```python
from build123d import *

# Parameters (mm, degrees)
SKETCH1_W           = 101.6
SKETCH1_H           = 101.6
SKETCH1_R           = 12.7
BOSS_EXTRUDE1_DEPTH = 3.175
SKETCH2_R           = 23.495
CUT_EXTRUDE1_DEPTH  = 5.08


with BuildPart() as part:
    # Sketch1 → Boss-Extrude1 (new body, symmetric)
    with BuildSketch(Plane(origin=(0, 0, 0), x_dir=(1, 0, 0), z_dir=(0, 1, 0))):
        Rectangle(SKETCH1_W, SKETCH1_H)
        with Locations((-31.75, 31.75)):
            Circle(SKETCH1_R, mode=Mode.SUBTRACT)
        with Locations((31.75, 31.75)):
            Circle(SKETCH1_R, mode=Mode.SUBTRACT)
    extrude(amount=BOSS_EXTRUDE1_DEPTH, both=True)

    # Sketch2 → Cut-Extrude1 (cut)
    with BuildSketch(Plane(origin=(0, 3.175, 0), x_dir=(1, 0, 0), z_dir=(0, 1, 0))):
        with Locations((-25.4, -10.318450471)):
            Circle(SKETCH2_R)
        with Locations((25.4, -10.318450471)):
            Circle(SKETCH2_R)
    extrude(amount=-CUT_EXTRUDE1_DEPTH, mode=Mode.SUBTRACT)


solid = part.part
```
Geometry check sheet. Reference: the model listing, model coordinates, mm. A direction names the side the tool comes from. Round coordinates to 2 decimals unless told otherwise and drop trailing zeros. Loops run counter-clockwise (first coordinate to the right, second up) from the corner with the lowest first, then second, coordinate; pieces in that order, holes last. Notation, with made-up numbers: (-14, 54) - (15, 54) arc R33 cw to (15, 91) - close; hole circle Ø9 at (8.25, 40.5). An arc over 180 degrees is marked (long way). Use a Markdown table: item, result.
Q1. Cross-section at A-A on z = -31.75. Record the cut outline in (x, y) (3 decimals), plus the area to 3 significant figures.
Solutions:
| item | result |
|---|---|
| outline | (-50.8, -3.175) - (-44.45, -3.175) - (-44.45, 3.175) - (-50.8, 3.175) - close; (-19.05, -3.175) - (19.05, -3.175) - (19.05, 3.175) - (-19.05, 3.175) - close; (44.45, -3.175) - (50.8, -3.175) - (50.8, 3.175) - (44.45, 3.175) - close |
| area | 323 mm2 |
Q2. Draft check along X on faces 1 (the flat face through (-1, 3.175, -1)), 2 (the flat face through (-50.8, 0, 1)), 3 (the cylindrical face through (8.08, 0.67, -5.56)). Enter one of: released by +X, released by -X, zero draft, split by the parting line, or undercut.
Solutions:
| item | result |
|---|---|
| face 1 | zero draft |
| face 2 | released by -X |
| face 3 | undercut |
Q3. Material ranges on line 1 (X direction, y = 0.75, z = -31); line 2 (Z direction, x = -31.75, y = -1.5); line 3 (X direction, y = 2.5, z = -29), recorded low to high.
Solutions:
| item | result |
|---|---|
| line 1 | x = -50.8 to -44.43, -19.07 to 19.07, 44.43 to 50.8 |
| line 2 | z = -50.8 to -44.45, -19.05 to -12.3, 32.94 to 50.8 |
| line 3 | x = -50.8 to -44.15, -19.35 to 19.35, 44.15 to 50.8 |
Q4. Cross-section at C-C on y = 0.75. Record the cut outline in (x, z) (3 decimals).
Solutions:
| item | result |
|---|---|
| outline | (-50.8, -50.8) - (50.8, -50.8) - (50.8, 50.8) - (-50.8, 50.8) - close; hole circle Ø46.99 at (-25.4, 10.318); hole circle Ø25.4 at (-31.75, -31.75); hole circle Ø46.99 at (25.4, 10.318); hole circle Ø25.4 at (31.75, -31.75) |
Q5. Access from +Z, -Z, +X, -X, +Y, -Y to the whole of each face (thin tool, end or side, straight path). Record for faces 4 (the cylindrical face through (-2.99, 0.67, 3.26)), 5 (the flat face through (-1, 0, 50.8)).
Solutions:
| item | result |
|---|---|
| face 4 | +Y |
| face 5 | +Z, +X, -X, +Y, -Y |
Q6. Cross-section at D-D on x = 41.5. Record the cut outline in (y, z) (3 decimals).
Solutions:
| item | result |
|---|---|
| outline | (-3.175, -50.8) - (3.175, -50.8) - (3.175, -39.888) - (-3.175, -39.888) - close; (-3.175, -23.612) - (3.175, -23.612) - (3.175, -6.793) - (-1.905, -6.793) - (-1.905, 27.43) - (3.175, 27.43) - (3.175, 50.8) - (-3.175, 50.8) - close |
Q7. Cross-section at B-B on x = -33. Record the cut outline in (y, z) (3 decimals).
Solutions:
| item | result |
|---|---|
| outline | (-3.175, -50.8) - (3.175, -50.8) - (3.175, -44.388) - (-3.175, -44.388) - close; (-3.175, -19.112) - (3.175, -19.112) - (3.175, -11.913) - (-1.905, -11.913) - (-1.905, 32.55) - (3.175, 32.55) - (3.175, 50.8) - (-3.175, 50.8) - close |
Q8. Go/stop test with flat-tipped pins: P1, Ø4, axis at x = 10.5, z = 4, coming from the +Y side (3 decimals); P2, Ø23.5, axis at x = -16.5, z = 0, coming from the +Y side (3 decimals). Record where each tip stops, or that it passes through.
Solutions:
| item | result |
|---|---|
| P1 | stops at y = -1.905 |
| P2 | stops at y = 3.175 |
